Autodesk Inventor part; units mm, degrees
ref_plane "YZ Plane" through (0, 0, 0) normal (1, 0, 0) x (0, 1, 0)
ref_plane "XZ Plane" through (0, 0, 0) normal (0, 1, 0) x (-1, 0, 0)
ref_plane "XY Plane" through (0, 0, 0) normal (0, 0, 1) x (1, 0, 0)
sketch "Sketch1" plane through (0, 0, 0) normal (0, 0, 1) x (1, 0, 0)
  line L0 (-10.9985, 0) -> (-5.4993, 9.525)
  line L1 (-5.4993, 9.525) -> (5.4993, 9.525)
  line L2 (5.4993, 9.525) -> (10.9985, 0)
  line L3 (10.9985, 0) -> (5.4993, -9.525)
  line L4 (5.4993, -9.525) -> (-5.4993, -9.525)
  line L5 (-5.4993, -9.525) -> (-10.9985, 0)
  point P0 (0, 0)
  point P1 (0, 0)
  dimension "d0" = 19.05
extrude "Extrusion1" add sketch "Sketch1" along normal blind 3.81
sketch "Sketch2" plane through (0, 0, 3.81) normal (0, 0, 1) x (1, 0, 0)
  circle A0 centre (0, 0) radius 6.35
  dimension "d3" = 12.7
extrude "Extrusion2" add sketch "Sketch2" along normal blind 63.5
thread "Thread1"
properties part number "LucasCharles Part 4 bolt to hold arm to wall mount Final" material "Stainless Steel, Austenitic"
For this review, take the finished solid that the model builds, in its own axes (mm). A direction names the side the tool comes from. Round coordinates to 2 decimals unless told otherwise and drop trailing zeros. Order: outer loops, then holes, each group sorted by start corner. A loop starts at its lowest first (then second) coordinate and runs counter-clockwise, first axis right, second up.
Q1. We need section C-C, the plane z = 24. Give the boundary of the cut face in (x, y), plus the area to 3 significant figures.
Findings below:
outline: circle Ø12.7 at (0, 0)
area: 127 mm2
Q2. We need section B-B, the plane y = 5.75. Give the boundary of the cut face in (x, z).
Findings below:
outline: (-7.68, 0) - (7.68, 0) - (7.68, 3.81) - (2.69, 3.81) - (2.69, 67.31) - (-2.69, 67.31) - (-2.69, 3.81) - (-7.68, 3.81) - close
Q3. We need section A-A, the plane x = 0. Give the boundary of the cut face in (y, z) (3 decimals).
Findings below:
outline: (-9.525, 0) - (9.525, 0) - (9.525, 3.81) - (6.35, 3.81) - (6.35, 67.31) - (-6.35, 67.31) - (-6.35, 3.81) - (-9.525, 3.81) - close
Q4. We need section D-D, the plane y = -8. Give the boundary of the cut face in (x, z).
Findings below:
outline: (-6.38, 0) - (6.38, 0) - (6.38, 3.81) - (-6.38, 3.81) - close
Q5. Insertion check: P1, Ø5, axis at x = -6.5, z = 46.5, coming from the -Y side; P2, Ø2, axis at y = -7.5, z = 31, coming from the +X side; P3, Ø10, axis at x = 2.5, z = 36.5, coming from the +Y side; P4, Ø6, axis at x = -3, y = 7.5, coming from the +Z side. Each pin has a flat end and moves straight along its axis. Give the tip position at first contact, or say it passes through.
Findings below:
P1: stops at y = -4.93
P2: passes through
P3: stops at y = 6.35
P4: stops at z = 67.31
Q6. Wall thickness on line 1 (Z direction, x = -5.75, y = 8.25); line 2 (Y direction, x = 2.75, z = 22); line 3 (Y direction, x = 1.5, z = 64.5): over which ranges is each line inside the solid? List them lowest first.
Findings below:
line 1: z = 0 to 3.81
line 2: y = -5.72 to 5.72
line 3: y = -6.17 to 6.17
Q7. Machinability: for faces 1 (the cylindrical face through (-1.38, 6.2, 35.12)), 2 (the flat face through (8.21, 4.83, 1.88)), which of the approach directions +Z, -Z, +X, -X, +Y, -Y give a long, thin tool a straight path to every point of the face, cutting with its end or side? Answer none if there is none.
Findings below:
face 1: +Z
face 2: +Z, -Z, +X, +Y
